from build123d import *

# Parameters (mm, degrees)
CUT_EXTRUDE_1_DEPTH = 48.531801986


with BuildPart() as part:
    # 草图1 → 旋转1 (revolve)
    with BuildSketch(Plane.XY, mode=Mode.PRIVATE) as revolve_1_sk:
        Polygon((0, 0), (0, 20.19), (2.5, 20.19), (2.5, 18.19), (23.5, 18.19), (23.5, 20.19), (26, 20.19), (26, 13.5), (38, 13.5), (38, 0), align=None)
    revolve(revolve_1_sk.sketch.rotate(Axis((0, 0, 0), (1, 0, 0)), 90), axis=Axis((0, 0, 0), (1, 0, 0)))

    # 草图2 → 切除-拉伸1 (cut, through all)
    with BuildSketch(Plane(origin=(38, 0, 0), x_dir=(0, 0, -1), z_dir=(1, 0, 0))):
        with BuildLine():
            Line((-2.5, -3.122498999), (-2.5, -6))
            Line((-2.5, -6), (2.5, -6))
            Line((2.5, -6), (2.5, -3.122498999))
            ThreePointArc((2.5, -3.122498999), (0, 4), (-2.5, -3.122498999))
        make_face()
    extrude(amount=-CUT_EXTRUDE_1_DEPTH, mode=Mode.SUBTRACT)


solid = part.part
Part model, mm, in its own coordinate system. A direction names the side the tool comes from. Coordinates: 2 decimals unless noted, no trailing zeros. Order: outer loops, then holes, each group sorted by start corner. A loop starts at its lowest first (then second) coordinate and runs counter-clockwise, first axis right, second up.
(1) Probe L1, parallel to Y at x = 21, z = 0; L2, parallel to X at y = -4, z = 18; L3, parallel to X at y = 16, z = 2. List the from-to ranges inside material, lowest first.
Check sheet entries:
L1: y = -18.19 to -6, 4 to 18.19
L2: x = 0 to 2.5, 23.5 to 26
L3: x = 0 to 26
(2) Pin check, flat tips, straight feed: pin 1 Ø4 at (x, z) = (25.5, -5) entering from +Y; pin 2 Ø2.5 at (x, y) = (12.5, -4) entering from +Z; pin 3 Ø6 at (x, z) = (29.5, 14) entering from +Y. Stop position of each tip, or through.
Check sheet entries:
pin 1: stops at y = 19.97
pin 2: stops at z = 17.98
pin 3: stops at y = 7.83
(3) Pull direction X, two halves, no side cores. Call faces 5 (the face through (0, 4.2, 0.3)), 6 (the face through (23.5, -8, 17)), 7 (the face through (19, 4, 0)): pulls with the +X half, pulls with the -X half, needs draft (parallel to the pull), parting line crosses it, or undercut.
Check sheet entries:
face 5: pulls with the -X half
face 6: undercut
face 7: needs draft
(4) Slice it at B-B, the plane y = -1.5. Write the cut outline in (x, z).
Check sheet entries:
outline: (0, -20.13) - (2.5, -20.13) - (2.5, -18.13) - (23.5, -18.13) - (23.5, -20.13) - (26, -20.13) - (26, -13.42) - (38, -13.42) - (38, -3.71) - (0, -3.71) - close; (0, 3.71) - (38, 3.71) - (38, 13.42) - (26, 13.42) - (26, 20.13) - (23.5, 20.13) - (23.5, 18.13) - (2.5, 18.13) - (2.5, 20.13) - (0, 20.13) - close
(5) Slice it at A-A, the plane z = 0. Write the cut outline in (x, y), and give its area (3 significant figures).
Check sheet entries:
outline: (0, -20.19) - (2.5, -20.19) - (2.5, -18.19) - (23.5, -18.19) - (23.5, -20.19) - (26, -20.19) - (26, -13.5) - (38, -13.5) - (38, -6) - (0, -6) - close; (0, 4) - (38, 4) - (38, 13.5) - (26, 13.5) - (26, 20.19) - (23.5, 20.19) - (23.5, 18.19) - (2.5, 18.19) - (2.5, 20.19) - (0, 20.19) - close
area: 910 mm2
(6) Tool access for faces 1 (the face through (19, -5, 2.5)), 2 (the face through (13.15, 16.14, 8.39)), 3 (the face through (26, 13.2, 4.2)), 4 (the face through (38, -3, 3)): list every direction of +Z, -Z, +X, -X, +Y, -Y with a clear straight run to the whole face (end or side of a thin tool).
Check sheet entries:
face 1: +X, -X
face 2: none
face 3: +X
face 4: +Z, -Z, +X, +Y, -Y
(7) Slice it at C-C, the plane x = 25. Write the cut outline in (y, z).
Check sheet entries:
outline: circle Ø40.38 at (0, 0); hole (-6, -2.5) - (-3.12, -2.5) arc R4 ccw (long way) to (-3.12, 2.5) - (-6, 2.5) - close
(8) Slice it at D-D, the plane z = 12. Write the cut outline in (x, y).
Check sheet entries:
outline: (0, -16.24) - (2.5, -16.24) - (2.5, -13.67) - (23.5, -13.67) - (23.5, -16.24) - (26, -16.24) - (26, -6.18) - (38, -6.18) - (38, 6.18) - (26, 6.18) - (26, 16.24) - (23.5, 16.24) - (23.5, 13.67) - (2.5, 13.67) - (2.5, 16.24) - (0, 16.24) - close
